Here's how the part is built. I have some questions about the finished solid (model axes, mm). Face numbers are marked on the shaded views. A direction names the side the tool comes from. Give positions to 0.01 mm unless a question says otherwise; leave off trailing zeros. Write each loop counter-clockwise with the first axis right and the second up, starting at its lowest first coordinate (ties: lowest second). Pieces come first, ordered by that corner, then holes. Notation, with made-up numbers: M 51.5,-30 L 76.5,-30 A19 cw 76.5,2 Z; hole C 69,37 d4. An arc over 180 degrees is marked long. Use one line per item in the form item = value. Start each with the question number.
from build123d import *

# Parameters (mm, degrees)
SKETCH_R           = 49
PAD_DEPTH          = 15
SKETCH001_R        = 5
POCKET_DEPTH       = 293.805591
POLARPATTERN_COUNT = 6
SKETCH002_R        = 25
PAD001_DEPTH       = 75
SKETCH003_R        = 17.5
POCKET001_DEPTH    = 30
SKETCH004_R        = 13
POCKET002_DEPTH    = 45
SKETCH005_R        = 6
SKETCH005_R_2      = 17.5
PAD002_DEPTH       = 15
SKETCH006_W        = 69.832336
SKETCH006_H        = 89.129906
POCKET003_DEPTH    = 60


with BuildPart() as part:
    # Sketch → Pad (new body)
    with BuildSketch(Plane.XZ):
        Circle(SKETCH_R)
    extrude(amount=PAD_DEPTH)

    # Sketch001 → Pocket (cut, through all)
    with BuildSketch(Plane.XZ.offset(15)):
        with Locations((0, 35)):
            Circle(SKETCH001_R)
    pocket = extrude(amount=-POCKET_DEPTH, mode=Mode.SUBTRACT)

    # PolarPattern: Pocket ×6 about axis
    polarpattern_axis = Axis((0, -15, 0), (0, -1, 0))
    for i in range(1, POLARPATTERN_COUNT):
        add(pocket.rotate(polarpattern_axis, i * 360 / POLARPATTERN_COUNT), mode=Mode.SUBTRACT)

    # Sketch002 → Pad001 (new body)
    with BuildSketch(Plane.XZ.offset(15)):
        Circle(SKETCH002_R)
    extrude(amount=PAD001_DEPTH)

    # Sketch003 → Pocket001 (cut)
    with BuildSketch(Plane.XZ.offset(90)):
        Circle(SKETCH003_R)
    extrude(amount=-POCKET001_DEPTH, mode=Mode.SUBTRACT)

    # Sketch004 → Pocket002 (cut)
    with BuildSketch(Plane.XZ.offset(60)):
        Circle(SKETCH004_R)
    extrude(amount=-POCKET002_DEPTH, mode=Mode.SUBTRACT)

    # Sketch005 → Pad002 (new body)
    with BuildSketch(Plane.XZ.offset(90)):
        with BuildLine():
            ThreePointArc((-28.618176, 9), (-30, 0), (-28.618176, -9))
            Line((-14.309088, -54.5), (-28.618176, -9))
            ThreePointArc((-14.309088, -54.5), (8e-06, -65), (14.309093, -54.499985))
            Line((14.309093, -54.499985), (28.618176, -9.000001))
            ThreePointArc((28.618176, -9.000001), (30, 0), (28.618176, 9))
            Line((14.309078, 54.50003), (28.618176, 9))
            ThreePointArc((14.309078, 54.50003), (-1.6e-05, 65), (-14.309088, 54.5))
            Line((-28.618176, 9), (-14.309088, 54.5))
        make_face()
        with Locations((0, 50)):
            Circle(SKETCH005_R, mode=Mode.SUBTRACT)
        with Locations((0, -50)):
            Circle(SKETCH005_R, mode=Mode.SUBTRACT)
        Circle(SKETCH005_R_2, mode=Mode.SUBTRACT)
    extrude(amount=-PAD002_DEPTH)

    # Sketch006 → Pocket003 (cut)
    with BuildSketch(Plane.XZ.offset(90)):
        with Locations((34.916168, 44.564953)):
            Rectangle(SKETCH006_W, SKETCH006_H)
    extrude(amount=-POCKET003_DEPTH, mode=Mode.SUBTRACT)


solid = part.part
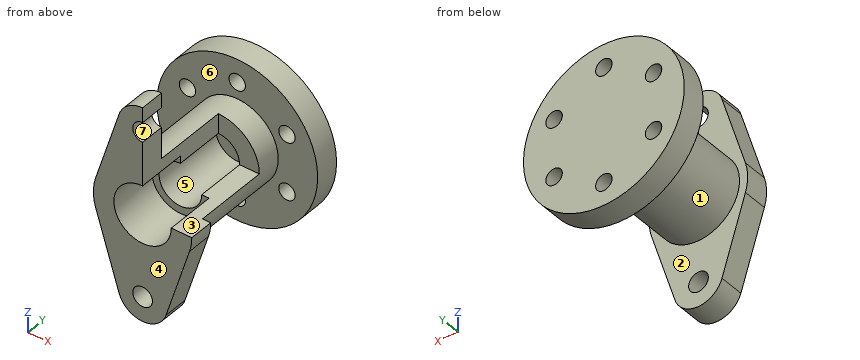
1) Suppose I cut it at D-D, the plane y = -11.5. List the corners of the cut face in (x, z) for me.
2) Thinking about a two-plate mould opening in Y: for the marked faces 1, 2, 3 and 4, which applies, released by +Y, released by -Y, zero draft, split by the parting line, or undercut?
3) Please list where these lines run through material, in increasing order: line 1 (Z direction, x = 0, y = -8); line 2 (Y direction, x = 9.5, z = -25); line 3 (Y direction, x = 16, z = -6).
4) Suppose I cut it at B-B, the plane z = 35. List the corners of the cut face in (x, y) for me.
5) On a 3-axis mill with a long thin cutter (end or side, diameter ignored), from which of +Z, -Z, +X, -X, +Y, -Y can I reach the whole of each face in a straight line? I mean the marked faces 5, 6 and 7. Say none if no direction works.
6) Suppose I cut it at A-A, the plane y = -25. List the corners of the cut face in (x, z) for me, and give its area (3 significant figures).
7) Will these pins go through, and if not, where does the flat tip stop? P1, Ø25, axis at y = -58.5, z = 24.5, coming from the +X side; P2, Ø12, axis at x = -19, y = -53, coming from the -Z side; P3, Ø12, axis at x = -27, y = -42, coming from the +Z side.
8) Suppose I cut it at C-C, the plane x = -7.5. List the corners of the cut face in (y, z) for me, and give its area (3 significant figures).
Checks:
q1.outline = C 0,0 d98; hole C -30.31,-17.5 d10; hole C -30.31,17.5 d10; hole C 0,-35 d10; hole C 0,35 d10; hole C 30.31,-17.5 d10; hole C 30.31,17.5 d10
q2.face_1 = undercut
q2.face_2 = undercut
q2.face_3 = zero draft
q2.face_4 = released by -Y
q3.line_1 = -49 to -40, -30 to 30, 40 to 49
q3.line_2 = -90 to -75, -15 to 0
q3.line_3 = -60 to 0
q4.outline = M -34.29,-15 L -5,-15 L -5,0 L -34.29,0 Z; M -20.44,-90 L 0,-90 L 0,-75 L -20.44,-75 Z; M 5,-15 L 34.29,-15 L 34.29,0 L 5,0 Z
q5.face_5 = -Y
q5.face_6 = none
q5.face_7 = +X, -Y
q6.outline = C 0,0 d50; hole C 0,0 d26
q6.area = 1,430 mm^2
q7.P1 = 0
q7.P2 = -21.35
q7.P3 = 13.56
q8.outline = M -90,-62.99 L -75,-62.99 L -75,-23.85 L -15,-23.85 L -15,-48.42 L 0,-48.42 L 0,48.42 L -15,48.42 L -15,23.85 L -75,23.85 L -75,62.99 L -90,62.99 L -90,15.81 L -60,15.81 L -60,10.62 L -15,10.62 L -15,-10.62 L -60,-10.62 L -60,-15.81 L -90,-15.81 Z
q8.area = 4,300 mm^2
